```python
from build123d import *

# Parameters (mm, degrees)
SKETCH_W              = 18.5
SKETCH_H              = 18.5
SKETCH_R              = 8.15
PAD_DEPTH             = 4
SKETCH001_W           = 18.5
SKETCH001_H           = 18.5
PAD001_DEPTH          = 3
SKETCH002_R           = 9.25
SKETCH003_R           = 5.4
SKETCH005_R           = 5.4
PAD002_DEPTH          = 2
CHAMFER_SIZE          = 1.5
CHAMFER001_SIZE       = 1.5
POCKET_DEPTH          = 112.426503
POLARPATTERN_COUNT    = 4
SKETCH007_R           = 4.4
SKETCH008_R           = 5.4
SKETCH009_R           = 5.4
PAD003_DEPTH          = 9
SKETCH010_R           = 4.4
POCKET001_DEPTH       = 5
POCKET002_DEPTH       = 131.363749
POLARPATTERN001_COUNT = 4
SKETCH012_W           = 6
SKETCH012_H           = 1
POCKET003_DEPTH       = 18.501


with BuildPart() as part:
    # Sketch → Pad (new body)
    with BuildSketch(Plane.XY):
        Rectangle(SKETCH_W, SKETCH_H)
        Circle(SKETCH_R, mode=Mode.SUBTRACT)
    extrude(amount=PAD_DEPTH)

    # Sketch001 (on Face7 of Pad) → Pad001 (join)
    with BuildSketch(Plane.XY.offset(4)):
        Rectangle(SKETCH001_W, SKETCH001_H)
    extrude(amount=PAD001_DEPTH)

    # Sketch002 (on Face10 of Pad001) → AdditiveLoft section 0
    with BuildSketch(Plane.XY.offset(7)):
        Circle(SKETCH002_R)
    # Sketch003 (on Face10 of Pad001) → AdditiveLoft section 1
    with BuildSketch(Plane.XY.offset(37)):
        Circle(SKETCH003_R)
    loft()

    # Sketch005 (on Face17 of AdditiveLoft) → Pad002 (join)
    with BuildSketch(Plane.XY.offset(37)):
        Circle(SKETCH005_R)
    extrude(amount=PAD002_DEPTH)

    # Chamfer
    chamfer_edges = [part.edges().sort_by_distance(p)[0] for p in [
        (-9.25, -9.25, 5.5),
        (-9.25, -9.25, 2),
        (9.25, -9.25, 5.5),
        (9.25, -9.25, 2),
        (9.25, 9.25, 2),
        (9.25, 9.25, 5.5),
        (-9.25, 9.25, 5.5),
        (-9.25, 9.25, 2),
    ]]
    chamfer(chamfer_edges, length=CHAMFER_SIZE)

    # Chamfer001
    chamfer001_edges = [part.edges().sort_by_distance(p)[0] for p in [
        (8.5, -8.5, 7),
        (-8.5, -8.5, 7),
        (-8.5, 8.5, 7),
        (8.5, 8.5, 7),
    ]]
    chamfer(chamfer001_edges, length=CHAMFER001_SIZE)

    # Sketch006 (on Face19 of Chamfer001) → Pocket (cut, through all)
    with BuildSketch(Plane.YZ.offset(9.25)):
        Polygon((0, 37), (-2.7, 7), (2.7, 7), align=None)
    pocket = extrude(amount=-POCKET_DEPTH, mode=Mode.SUBTRACT)

    # PolarPattern: Pocket ×4 about axis
    polarpattern_axis = Axis((0, 0, 0), (0, 0, 1))
    for i in range(1, POLARPATTERN_COUNT):
        add(pocket.rotate(polarpattern_axis, i * 360 / POLARPATTERN_COUNT), mode=Mode.SUBTRACT)

    # Sketch007 (on Face47 of PolarPattern) → AdditiveLoft001 section 0
    with BuildSketch(Plane.XY.offset(39)):
        Circle(SKETCH007_R)
    # Sketch008 → AdditiveLoft001 section 1
    with BuildSketch(Plane.XY.offset(41)):
        Circle(SKETCH008_R)
    loft()

    # Sketch009 (on Face56 of AdditiveLoft001) → Pad003 (join)
    with BuildSketch(Plane.XY.offset(41)):
        Circle(SKETCH009_R)
    extrude(amount=PAD003_DEPTH)

    # Sketch010 (on Face57 of Pad003) → Pocket001 (cut)
    with BuildSketch(Plane.XY.offset(50)):
        Circle(SKETCH010_R)
    extrude(amount=-POCKET001_DEPTH, mode=Mode.SUBTRACT)

    # Sketch011 (on Face26 of Pocket001) → Pocket002 (cut, through all)
    with BuildSketch(Plane.YZ.offset(9.25)):
        Polygon((-3, 50), (3, 50), (0.85, 45), (-0.85, 45), align=None)
    pocket002 = extrude(amount=-POCKET002_DEPTH, mode=Mode.SUBTRACT)

    # PolarPattern001: Pocket002 ×4 about axis
    polarpattern001_axis = Axis((0, 0, 0), (0, 0, 1))
    for i in range(1, POLARPATTERN001_COUNT):
        add(pocket002.rotate(polarpattern001_axis, i * 360 / POLARPATTERN001_COUNT), mode=Mode.SUBTRACT)

    # Sketch012 (on Face4 of PolarPattern001) → Pocket003 (cut, through all)
    with BuildSketch(Plane(origin=(0, 9.25, 0), x_dir=(-1, 0, 0), z_dir=(0, 1, 0))):
        with Locations((0, 43)):
            Rectangle(SKETCH012_W, SKETCH012_H)
    extrude(amount=-POCKET003_DEPTH, mode=Mode.SUBTRACT)


solid = part.part
```
CAD build for the part. Positions are in the model's coordinates, mm. A direction names the side the tool comes from. Coordinates: 2 decimals unless noted, no trailing zeros. Write each loop counter-clockwise with the first axis right and the second up, starting at its lowest first coordinate (ties: lowest second). Pieces come first, ordered by that corner, then holes. Notation, with made-up numbers: (53.25, 63) -> (99.25, 63) arc R33 ccw to (99.25, 99) -> close; hole circle Ø1 at (52.25, 13.25). An arc over 180 degrees is marked (long way). Return JSON: item names as keys, results as strings. Group by question number.
Q1. Cut at A-A, the plane z = 32.5. Give the cut face in (x, y) (1 decimal), then the cut area to 3 significant figures.
Q2. Drill centre lines: line 1 (Y direction, x = 0, z = 2.4); line 2 (X direction, y = 1.25, z = 29); line 3 (X direction, y = 5.75, z = 20.5) (3 decimals). Where is each one in solid material? Low to high.
Q3. Cut at B-B, the plane y = 2. State how many separate pieces and enclosed holes the cut face has, then the cut area to 3 significant figures.
Q4. Flat gauge pins, fed straight in: pin 1 (2 mm diameter, centred on y = 5.5, z = 14.5, fed in from +X); pin 2 (6.5 mm diameter, centred on x = 1, y = -2.5, fed in from -Z); pin 3 (3 mm diameter, centred on y = 5, z = 16, fed in from +X); pin 4 (2 mm diameter, centred on y = 6.5, z = 44.5, fed in from +X). Where does each tip first touch, or does it go through?
Q5. Pull direction X, two halves, no side cores. Call faces 1 (the face through (0, 0, 45)), 2 (the face through (4.988, -2.068, 44.437)), 3 (the face through (-4.5, -1.91, 47.47)): released by +X, released by -X, zero draft, split by the parting line, or undercut.
Q6. Which spindle directions (+Z, -Z, +X, -X, +Y, -Y) get a long thin tool onto all of the face, cutting with end or side? Do faces 4 (the face through (5.22, 5.1, 22.21)), 5 (the face through (-3.085, 3.137, 46.979)), 6 (the face through (0, 0, 7)), 7 (the face through (3, 0, 43)), 8 (the face through (-4.496, 1.94, 47.535)). Say none if no direction does.
Q7. Cut at C-C, the plane z = 13.5. Give the cut face in (x, y) (3 decimals).
Returned:
{
 "1": {"outline": "(-6, -0.4) arc R6 ccw to (-0.4, -6) -> (-0.4, -0.4) -> close; (-6, 0.4) -> (-0.4, 0.4) -> (-0.4, 6) arc R6 ccw to start; (0.4, -6) arc R6 ccw to (6, -0.4) -> (0.4, -0.4) -> close; (0.4, 0.4) -> (6, 0.4) arc R6 ccw to (0.4, 6) -> close", "area": "93.6 mm2"},
 "2": {"line 1": "y = -9.25 to -8.15, 8.15 to 9.25", "line 2": "x = -6.3 to -0.72, 0.72 to 6.3", "line 3": "x = -4.843 to -1.485, 1.485 to 4.843"},
 "3": {"separate pieces": "2", "enclosed holes": "1", "area": "390 mm2"},
 "4": {"pin 1": "stops at x = 6.98", "pin 2": "stops at z = 4", "pin 3": "stops at x = 7.33", "pin 4": "passes through"},
 "5": {"face 1": "undercut", "face 2": "split by the parting line", "face 3": "zero draft"},
 "6": {"face 4": "+Z, +X, +Y", "face 5": "+Z", "face 6": "none", "face 7": "+Y, -Y", "face 8": "+Z, +X, -X"},
 "7": {"outline": "(-8.146, -2.115) arc R8.416 ccw to (-2.115, -8.146) -> (-2.115, -2.115) -> close; (-8.146, 2.115) -> (-2.115, 2.115) -> (-2.115, 8.146) arc R8.416 ccw to start; (2.115, -8.146) arc R8.416 ccw to (8.146, -2.115) -> (2.115, -2.115) -> close; (2.115, 2.115) -> (8.146, 2.115) arc R8.416 ccw to (2.115, 8.146) -> close"}
}
